from build123d import *

# Parameters (mm, degrees)
CROQUIS11_R             = 62
CROQUIS11_R_2           = 20
SALIENTE_EXTRUIR3_DEPTH = 8
CROQUIS15_R             = 21.5
CORTAR_EXTRUIR4_DEPTH   = 89.045442812
CROQUIS16_R             = 23.5
CORTAR_EXTRUIR5_DEPTH   = 4
CROQUIS21_R             = 62
CROQUIS21_R_2           = 52.5
CORTAR_EXTRUIR10_DEPTH  = 5


with BuildPart() as part:
    # Croquis11 → Saliente-Extruir3 (new body)
    with BuildSketch(Plane(origin=(0, 0, 0), x_dir=(0, 0, -1), z_dir=(1, 0, 0))):
        Circle(CROQUIS11_R)
        Circle(CROQUIS11_R_2, mode=Mode.SUBTRACT)
    extrude(amount=-SALIENTE_EXTRUIR3_DEPTH)

    # Croquis15 → Cortar-Extruir4 (cut, through all)
    with BuildSketch(Plane(origin=(0, 0, 0), x_dir=(0, 0, -1), z_dir=(1, 0, 0))):
        Circle(CROQUIS15_R)
    extrude(amount=-CORTAR_EXTRUIR4_DEPTH, mode=Mode.SUBTRACT)

    # Croquis16 → Cortar-Extruir5 (cut)
    with BuildSketch(Plane.ZY.offset(8)):
        Circle(CROQUIS16_R)
    extrude(amount=-CORTAR_EXTRUIR5_DEPTH, mode=Mode.SUBTRACT)

    # Croquis21 → Cortar-Extruir10 (cut)
    with BuildSketch(Plane(origin=(0, 0, 0), x_dir=(0, 0, -1), z_dir=(1, 0, 0))):
        Circle(CROQUIS21_R)
        Circle(CROQUIS21_R_2, mode=Mode.SUBTRACT)
    extrude(amount=-CORTAR_EXTRUIR10_DEPTH, mode=Mode.SUBTRACT)


solid = part.part
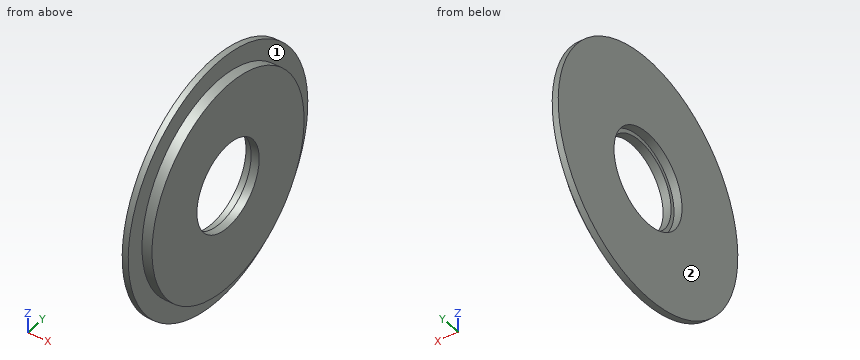
Model file for the job. Use its own axes, mm. Face numbers are marked on the shaded views. A direction names the side the tool comes from. Give positions to 0.01 mm unless a question says otherwise; leave off trailing zeros. Loops run counter-clockwise (first coordinate to the right, second up) from the corner with the lowest first, then second, coordinate; pieces in that order, holes last.
1) Saw through at D-D (x = -6.75). Write the cut outline in (y, z), plus the area to 3 significant figures.
2) Tool access for the marked faces 1 and 2: list every direction of +Z, -Z, +X, -X, +Y, -Y with a clear straight run to the whole face (end or side of a thin tool).
3) Flat gauge pins, fed straight in: pin 1 Ø1.5 at (x, z) = (-3, 22) entering from +Y; pin 2 Ø1 at (x, z) = (-1, 0) entering from +Y. Where does each tip first touch, or does it go through?
4) Wall check: line 1 (Y direction, x = -6.85, z = 0); line 2 (Y direction, x = -1, z = 0); line 3 (X direction, y = 7.5, z = -53.5). Give the ranges that are in metal, low to high.
5) Saw through at C-C (z = 43.5). Write the cut outline in (x, y), plus the area to 3 significant figures.
6) Saw through at A-A (y = 0). Write the cut outline in (x, z).
Answer block:
1. outline: circle Ø124 at (0, 0); hole circle Ø47 at (0, 0)
1. area: 10,300 mm2
2. face 1: +X
2. face 2: +Z, -Z, -X, +Y, -Y
3. pin 1: stops at y = 48.01
3. pin 2: stops at y = 52.5
4. line 1: y = -62 to -23.5, 23.5 to 62
4. line 2: y = -52.5 to -21.5, 21.5 to 52.5
4. line 3: x = -8 to -5
5. outline: (-8, -44.18) - (-5, -44.18) - (-5, -29.39) - (0, -29.39) - (0, 29.39) - (-5, 29.39) - (-5, 44.18) - (-8, 44.18) - close
5. area: 559 mm2
6. outline: (-8, -62) - (-5, -62) - (-5, -52.5) - (0, -52.5) - (0, -21.5) - (-4, -21.5) - (-4, -23.5) - (-8, -23.5) - close; (-8, 23.5) - (-4, 23.5) - (-4, 21.5) - (0, 21.5) - (0, 52.5) - (-5, 52.5) - (-5, 62) - (-8, 62) - close
